Design review of the part shown in the three views and the two pictorial views. Dimensions are in mm from the part's minimum x, y and z. Give positions to 0.01 mm unless a question says otherwise; leave off trailing zeros. Write each loop counter-clockwise with the first axis right and the second up, starting at its lowest first coordinate (ties: lowest second). Pieces come first, ordered by that corner, then holes. Notation, with made-up numbers: M -22,-11 L 8,-11 A22 cw 8,23 Z; hole C -30,55.25 d10. An arc over 180 degrees is marked long. Write item = value, one per line.
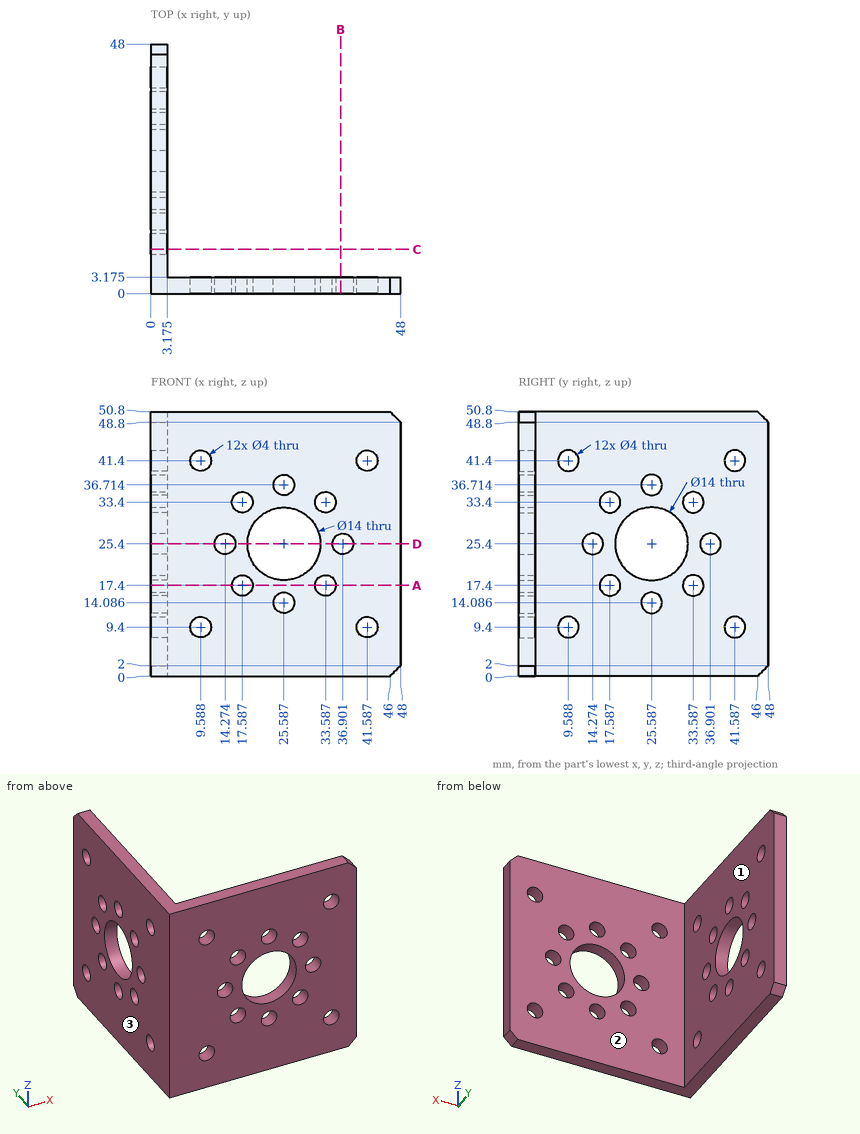
1. For line 1 along Y through (x, z) = (1.35, 41.4); line 2 along Y through (x, z) = (29.5, 14) (1 decimal), list the stretches that pass through material, from the lowest coordinate up. Write a range as from..to.
Responses:
line_1 = 0..7.59, 11.59..39.59, 43.59..48
line_2 = 0..3.2
2. The part is to be moulded in two halves that separate along X. For the marked faces 1, 2 and 3, say which applies: +X half, -X half, draft (parallel to the pull), parting line (faces both ways), or undercut.
Responses:
face_1 = +X half
face_2 = draft
face_3 = -X half
3. We need section C-C, the plane y = 8.5. Write out the cut boundary in (x, z) (1 decimal).
Responses:
outline = M 0,0 L 3.2,0 L 3.2,7.7 L 0,7.7 Z; M 0,11.1 L 3.2,11.1 L 3.2,39.7 L 0,39.7 Z; M 0,43.1 L 3.2,43.1 L 3.2,50.8 L 0,50.8 Z
4. We need section D-D, the plane z = 25.4. Count the separate pieces of the cut face and the enclosed holes in it, then the cut area to 3 significant figures.
Responses:
separate_pieces = 7
enclosed_holes = 0
area = 155 mm2
5. Insertion check: P1, Ø1.5, axis at y = 15.5, z = 45, coming from the +X side (1 decimal); P2, Ø5, axis at x = 17.59, z = 17.4, coming from the +Y side (1 decimal). Each pin has a flat end and moves straight along its axis. Give the tip position at first contact, or say it passes through.
Responses:
P1 = 3.2
P2 = 3.2
6. We need section B-B, the plane x = 36.5. Write out the cut boundary in (y, z) (1 decimal).
Responses:
outline = M 0,0 L 3.2,0 L 3.2,23.4 L 0,23.4 Z; M 0,27.4 L 3.2,27.4 L 3.2,50.8 L 0,50.8 Z
7. We need section A-A, the plane z = 17.4. Write out the cut boundary in (x, y) (1 decimal), then the cut area to 3 significant figures.
Responses:
outline = M 0,0 L 15.6,0 L 15.6,3.2 L 3.2,3.2 L 3.2,15.6 L 0,15.6 Z; M 0,19.6 L 3.2,19.6 L 3.2,31.6 L 0,31.6 Z; M 0,35.6 L 3.2,35.6 L 3.2,48 L 0,48 Z; M 19.6,0 L 31.6,0 L 31.6,3.2 L 19.6,3.2 Z; M 35.6,0 L 48,0 L 48,3.2 L 35.6,3.2 Z
area = 244 mm2
